from build123d import *

# Parameters (mm, degrees)
SKETCH1_W           = 63.5
SKETCH1_H           = 32.766
SKETCH1_R           = 2.2225
SKETCH1_W_2         = 10.16
SKETCH1_H_2         = 3.175
SKETCH1_W_3         = 40.64
SKETCH1_H_3         = 19.431
BOSS_EXTRUDE2_DEPTH = 3.175


with BuildPart() as part:
    # Sketch1 → Boss-Extrude2 (new body)
    with BuildSketch(Plane(origin=(0, 0, 0), x_dir=(1, 0, 0), z_dir=(0, 1, 0))):
        with Locations((0, 1.5875)):
            Rectangle(SKETCH1_W, SKETCH1_H)
        with Locations(Location((-24.4475, 5.711910092, 0), (0, 0, 270))):
            Circle(SKETCH1_R, mode=Mode.SUBTRACT)
        with Locations(Location((-24.4475, -4.93498923, 0), (0, 0, 270))):
            Circle(SKETCH1_R, mode=Mode.SUBTRACT)
        with Locations(Location((24.4475, 5.711910092, 0), (0, 0, 270))):
            Circle(SKETCH1_R, mode=Mode.SUBTRACT)
        with Locations(Location((24.4475, -4.93498923, 0), (0, 0, 270))):
            Circle(SKETCH1_R, mode=Mode.SUBTRACT)
        with Locations((21.59, 13.843)):
            Rectangle(SKETCH1_W_2, SKETCH1_H_2, mode=Mode.SUBTRACT)
        with Locations((1.27, 13.843)):
            Rectangle(SKETCH1_W_2, SKETCH1_H_2, mode=Mode.SUBTRACT)
        with Locations((-19.05, 13.843)):
            Rectangle(SKETCH1_W_2, SKETCH1_H_2, mode=Mode.SUBTRACT)
        Rectangle(SKETCH1_W_3, SKETCH1_H_3, mode=Mode.SUBTRACT)
    extrude(amount=BOSS_EXTRUDE2_DEPTH)


solid = part.part
Model file for the job. Use its own axes, mm. A direction names the side the tool comes from. Coordinates: 2 decimals unless noted, no trailing zeros. Order: outer loops, then holes, each group sorted by start corner. A loop starts at its lowest first (then second) coordinate and runs counter-clockwise, first axis right, second up. Notation, with made-up numbers: (85, -30) -> (104, -30) arc R33 ccw to (104, 5) -> close; hole circle Ø4 at (-37, 42.5). An arc over 180 degrees is marked (long way). Return JSON: item names as keys, results as strings. Group by question number.
Item 1: Tool access for faces 1 (the flat face through (20.32, 2, 0)), 2 (the flat face through (31.75, 2, -1)): list every direction of +Z, -Z, +X, -X, +Y, -Y with a clear straight run to the whole face (end or side of a thin tool).
Item 2: Saw through at C-C on y = 2.2. State how many separate pieces and enclosed holes the cut face has, then the cut area to 3 significant figures.
Item 3: Wall check: line 1 along X through (y, z) = (2.65, -13); line 2 along X through (y, z) = (1.4, -5.5); line 3 along Z through (x, y) = (-18, 1.65). Give the ranges that are in metal, low to high. Write a range as [from, to].
Item 4: Saw through at B-B on x = -18.5. Write the cut outline in (y, z) (1 decimal).
Item 5: Pull direction Z, two halves, no side cores. Call faces 3 (the flat face through (0, 2, 9.716)), 4 (the flat face through (0, 2, -17.97)), 5 (the flat face through (7, 3.175, -13)): pulls with the +Z half, pulls with the -Z half, needs draft (parallel to the pull), parting line crosses it, or undercut.
Item 6: Flat gauge pins, fed straight in: P1, Ø4, axis at x = 24.45, z = 4.93, coming from the +Y side; P2, Ø6, axis at x = -22.5, z = -5.5, coming from the -Y side. Where does each tip first touch, or does it go through?
Item 7: Saw through at A-A on x = 7.5. Write the cut outline in (y, z) (1 decimal), then the cut area to 3 significant figures.
Values found:
{
 "1": {"face 1": "+Y, -Y", "face 2": "+Z, -Z, +X, +Y, -Y"},
 "2": {"separate pieces": "1", "enclosed holes": "8", "area": "1,130 mm2"},
 "3": {"line 1": "x = [-31.75, -24.13], [-13.97, -3.81], [6.35, 16.51], [26.67, 31.75]", "line 2": "x = [-31.75, -26.66], [-22.24, -20.32], [20.32, 22.24], [26.66, 31.75]", "line 3": "z = [-17.97, -15.43], [-12.26, -9.72], [9.72, 14.8]"},
 "4": {"outline": "(0, -18) -> (3.2, -18) -> (3.2, -15.4) -> (0, -15.4) -> close; (0, -12.3) -> (3.2, -12.3) -> (3.2, -9.7) -> (0, -9.7) -> close; (0, 9.7) -> (3.2, 9.7) -> (3.2, 14.8) -> (0, 14.8) -> close"},
 "5": {"face 3": "undercut", "face 4": "pulls with the -Z half", "face 5": "needs draft"},
 "6": {"P1": "passes through", "P2": "stops at y = 0"},
 "7": {"outline": "(0, -18) -> (3.2, -18) -> (3.2, -9.7) -> (0, -9.7) -> close; (0, 9.7) -> (3.2, 9.7) -> (3.2, 14.8) -> (0, 14.8) -> close", "area": "42.3 mm2"}
}
